Source: CAD feature listing. Evaluate the final solid. Frame: model axes, mm. Coordinates: 2 decimals unless noted, no trailing zeros. Write each loop counter-clockwise with the first axis right and the second up, starting at its lowest first coordinate (ties: lowest second). Pieces come first, ordered by that corner, then holes. Notation, with made-up numbers: M 0,-29 L 5,-29 A15 cw 5,-14 Z; hole C 5.25,-2 d6. An arc over 180 degrees is marked long. One line per item, written item: value. Start each with the question number.
Item 1: Cut plane A-A, the plane x = 0. Output: boundary loops of the cut face in (y, z).
Item 2: Ray query, L1, parallel to Z at x = 0, y = 0.8; L2, parallel to X at y = 0.4, z = 0; L3, parallel to Z at x = -0.5, y = 0.9. Return the intervals inside material, ascending. Write a range as from..to.
Item 3: Cut plane B-B, the plane z = 0.6. Output: boundary loops of the cut face in (x, y).
Item 4: Mould query, pull axis Z, two halves, no side actions, for faces 1 (the cylindrical face through (1.2, 0.99, 0.05)), 2 (the cylindrical face through (0, 1, 1)). Classes: released by +Z, released by -Z, zero draft, split by the parting line, or undercut.
Item 5: Cut plane D-D, the plane x = -9. Output: boundary loops of the cut face in (y, z) (3 decimals), then the cut area to 3 significant figures.
Item 6: Cut plane C-C, the plane y = 0.9. Output: boundary loops of the cut face in (x, z), then the cut area to 3 significant figures.
```python
from build123d import *

# Parameters (mm, degrees)
SKETCH1_R           = 1.2
SKETCH1_R_2         = 1
BOSS_EXTRUDE1_DEPTH = 2
BOSS_EXTRUDE3_DEPTH = 0.25
SKETCH3_OUTSIDE_W   = 6.938
SKETCH3_OUTSIDE_H   = 6.538
CUT_EXTRUDE3_DEPTH  = 9.9


with BuildPart() as part:
    # Sketch1 → Boss-Extrude1 (new body)
    with BuildSketch(Plane(origin=(0, 0, 0), x_dir=(1, 0, 0), z_dir=(0, 1, 0))):
        Circle(SKETCH1_R)
        Circle(SKETCH1_R_2, mode=Mode.SUBTRACT)
    extrude(amount=BOSS_EXTRUDE1_DEPTH)

    # Sketch2 → Boss-Extrude3 (add)
    with BuildSketch(Plane(origin=(0, 2, 0), x_dir=(1, 0, 0), z_dir=(0, 1, 0))):
        with BuildLine():
            Line((-11.094706331, -0.25), (-1.173669459, -0.25))
            ThreePointArc((-1.173669459, -0.25), (-1.2, 0), (-1.173669459, 0.25))
            Line((-1.173669459, 0.25), (-11.094706331, 0.25))
            Line((-11.094706331, 0.25), (-11.094706331, -0.25))
        make_face()
    extrude(amount=-BOSS_EXTRUDE3_DEPTH)

    # Sketch3 outside → Cut-Extrude3 (cut)
    with BuildSketch(Plane.ZY.offset(11.094706331)):
        with Locations((0, 1)):
            Rectangle(SKETCH3_OUTSIDE_W, SKETCH3_OUTSIDE_H)
        Polygon((-0.25, 1.875), (0, 2), (0.25, 1.875), (0, 1.75), align=None, mode=Mode.SUBTRACT)
    extrude(amount=-CUT_EXTRUDE3_DEPTH, mode=Mode.SUBTRACT)


solid = part.part
```
From the geometry:
1. outline: M 0,-1.2 L 2,-1.2 L 2,-1 L 0,-1 Z; M 0,1 L 2,1 L 2,1.2 L 0,1.2 Z
2. L1: z = -1.2..-1, 1..1.2
2. L2: x = -1.19..-1, 1..1.2
2. L3: z = -1.09..-0.87, 0.87..1.09
3. outline: M -1.04,0 L -0.8,0 L -0.8,2 L -1.04,2 Z; M 0.8,0 L 1.04,0 L 1.04,2 L 0.8,2 Z
4. face 1: split by the parting line
4. face 2: undercut
5. outline: M 1.75,0 L 1.875,-0.25 L 2,0 L 1.875,0.25 Z
5. area: 0.0625 mm²
6. outline: M -1.19,-0.11 A1.2 ccw long -1.19,0.11 Z; hole C 0,0 d2
6. area: 1.38 mm²
